Print and shaded views of the part. All mm, measured from the part's lowest x, y and z. A direction names the side the tool comes from. Coordinates: 2 decimals unless noted, no trailing zeros. Order: outer loops, then holes, each group sorted by start corner. A loop starts at its lowest first (then second) coordinate and runs counter-clockwise, first axis right, second up. Notation, with made-up numbers: (-26.75, 89) -> (1.25, 89) arc R23 cw to (1.25, 122) -> close; hole circle Ø7 at (57.25, 67.5). An arc over 180 degrees is marked (long way). Write item = value, one per line. Start each with the question number.
Q1. Cut at C-C, the plane x = 31. List the corners of the cut face in (y, z).
Q2. Mould opens along Y. For the marked faces 1, 2 and 3 say: +Y half, -Y half, draft (parallel to the pull), parting line (faces both ways), or undercut.
Q3. Flat gauge pins, fed straight in: pin 1 (15 mm diameter, centred on y = 29.5, z = 27, fed in from +X) (1 decimal); pin 2 (15 mm diameter, centred on x = 77.79, y = 31.75, fed in from -Z); pin 3 (3 mm diameter, centred on y = 33.5, z = 3, fed in from +X). Where does each tip first touch, or does it go through?
Q4. Wall check: line 1 (X direction, y = 31, z = 12); line 2 (Y direction, x = 78, z = 10.5); line 3 (X direction, y = 48.5, z = 25) (1 decimal). Give the ranges that are in metal, low to high. Write a range as from..to.
Q5. Cut at B-B, the plane z = 24. List the corners of the cut face in (x, y) (1 decimal).
Q6. 3-axis set-ups, long thin cutter, end or side, ignore diameter. For the marked faces 4, 5, 6 and 7: which of +Z, -Z, +X, -X, +Y, -Y reach the whole face in a straight line?
Q7. Cut at A-A, the plane y = 31.75. Give the number of separate pieces and of enclosed holes in the cut face, plus the area to 3 significant figures.
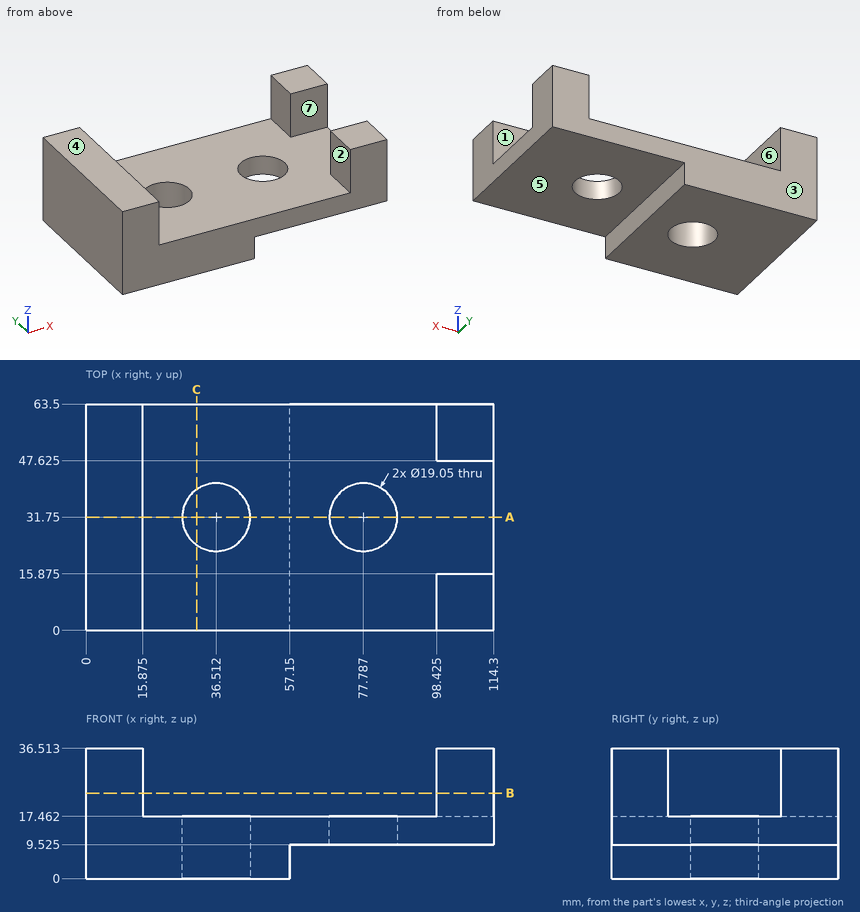
Here are the results:
q1.outline = (0, 0) -> (23.98, 0) -> (23.98, 17.46) -> (0, 17.46) -> close; (39.52, 0) -> (63.5, 0) -> (63.5, 17.46) -> (39.52, 17.46) -> close
q2.face_1 = undercut
q2.face_2 = draft
q2.face_3 = +Y half
q3.pin_1 = 15.9
q3.pin_2 = through
q3.pin_3 = 57.15
q4.line_1 = 0..27.02, 46.01..68.29, 87.28..114.3
q4.line_2 = 0..22.23, 41.27..63.5
q4.line_3 = 0..15.9, 98.4..114.3
q5.outline = (0, 0) -> (15.9, 0) -> (15.9, 63.5) -> (0, 63.5) -> close; (98.4, 0) -> (114.3, 0) -> (114.3, 15.9) -> (98.4, 15.9) -> close; (98.4, 47.6) -> (114.3, 47.6) -> (114.3, 63.5) -> (98.4, 63.5) -> close
q6.face_4 = +Z, +X, -X, +Y, -Y
q6.face_5 = -Z, +X, +Y, -Y
q6.face_6 = +Z, +Y, -Y
q6.face_7 = +Z, +X
q7.separate_pieces = 3
q7.enclosed_holes = 0
q7.area = 1,270 mm²
